```python
from build123d import *

# Parameters (mm, degrees)
F1_DEPTH = 200
F2_R     = 2
F4_DEPTH = 2
F6_D     = 5
F6_DEPTH = 2


with BuildPart() as f1:
    # F0 (on Front) → F1 (new body)
    with BuildSketch(Plane.XZ):
        Polygon((35, 0), (0, 0), (0, -345), (28, -345), (28, -295), (8, -271.164928), (8, -191.164928), (30, -130.720425), (30, -80.720425), (28, -80.720425), (28, -130.367771), (6, -190.812274), (6, -271.892869), (26, -295.72794), (26, -343), (2, -343), (2, -2), (33, -2), (33, -23), (35, -23), align=None)
    extrude(amount=F1_DEPTH)

    # F2
    f2_edges = [f1.edges().sort_by_distance(p)[0] for p in [
        (0, -100, 0),
        (35, -100, 0),
        (33, -100, -2),
        (2, -100, -2),
        (0, -100, -345),
        (2, -100, -343),
        (28, -100, -345),
        (26, -100, -343),
        (26, -100, -295.72794),
        (28, -100, -295),
        (8, -100, -271.164928),
        (6, -100, -271.892869),
        (6, -100, -190.812274),
        (8, -100, -191.164928),
        (30, -100, -130.720425),
        (28, -100, -130.367771),
    ]]
    fillet(f2_edges, radius=F2_R)

    # F3 (on face) → F4 (cut)
    with BuildSketch(Plane(origin=(0, 0, 0), x_dir=(0, -1, 0), z_dir=(-1, 0, 0))):
        with BuildLine():
            Line((70, -50), (30, -50))
            ThreePointArc((30, -50), (26.464466, -51.464466), (25, -55))
            Line((25, -55), (25, -290))
            ThreePointArc((25, -290), (26.464466, -293.535534), (30, -295))
            Line((30, -295), (70, -295))
            ThreePointArc((70, -295), (73.535534, -293.535534), (75, -290))
            Line((75, -290), (75, -55))
            ThreePointArc((75, -55), (73.535534, -51.464466), (70, -50))
        make_face()
        with BuildLine():
            ThreePointArc((175, -55), (173.535534, -51.464466), (170, -50))
            Line((170, -50), (130, -50))
            ThreePointArc((130, -50), (126.464466, -51.464466), (125, -55))
            Line((125, -55), (125, -290))
            ThreePointArc((125, -290), (126.464466, -293.535534), (130, -295))
            Line((130, -295), (170, -295))
            ThreePointArc((170, -295), (173.535534, -293.535534), (175, -290))
            Line((175, -290), (175, -55))
        make_face()
    extrude(amount=-F4_DEPTH, mode=Mode.SUBTRACT)

    # F6
    with Locations(Plane(origin=(28, 0, 0), x_dir=(0, -1, 0), z_dir=(-1, 0, 0))):
        with Locations((50, -105.367771), (150, -105.367771)):
            Hole(F6_D / 2, depth=F6_DEPTH)


solid = f1.part
```
For this review, take the finished solid that the model builds, in its own axes (mm). A direction names the side the tool comes from. Coordinates: 2 decimals unless noted, no trailing zeros. Write each loop counter-clockwise with the first axis right and the second up, starting at its lowest first coordinate (ties: lowest second). Pieces come first, ordered by that corner, then holes. Notation, with made-up numbers: (-5.75, 3.25) -> (34.25, 3.25) arc R27 ccw to (34.25, 31.25) -> close; hole circle Ø1 at (18.25, 65.25). An arc over 180 degrees is marked (long way). Put each result on its own line as item: value.
Q1. Wall thickness on L1, parallel to X at y = -106, z = -209; L2, parallel to X at y = -91, z = -115.5; L3, parallel to Z at x = 31, y = -85.5: over which ranges is each line inside the solid? List them lowest first.
From the geometry:
L1: x = 0 to 2, 6 to 8
L2: x = 0 to 2, 28 to 30
L3: z = -2 to 0
Q2. Take a section at B-B, the plane x = 17. State the section outline as (y, z) points.
From the geometry:
outline: (-200, -345) -> (0, -345) -> (0, -343) -> (-200, -343) -> close; (-200, -285) -> (0, -285) -> (0, -281.89) -> (-200, -281.89) -> close; (-200, -166.44) -> (0, -166.44) -> (0, -160.59) -> (-200, -160.59) -> close; (-200, -2) -> (0, -2) -> (0, 0) -> (-200, 0) -> close
Q3. The part is to be moulded in two halves that separate along Z. For faces 1 (the flat face through (14, -99, -345)), 2 (the flat face through (17.152, -98.6, -160.172)), 3 (the flat face through (0, -99, -170)), say which applies: +Z half, -Z half, draft (parallel to the pull), parting line (faces both ways), or undercut.
From the geometry:
face 1: -Z half
face 2: undercut
face 3: draft
Q4. Take a section at A-A, the plane z = -307.5. State the section outline as (x, y) points, then the cut area to 3 significant figures.
From the geometry:
outline: (0, -200) -> (2, -200) -> (2, 0) -> (0, 0) -> close; (26, -200) -> (28, -200) -> (28, 0) -> (26, 0) -> close
area: 800 mm2
Q5. Clearance check with flat-ended pins moving along their axes: pin 1 Ø10 at (y, z) = (-102, -248.5) entering from +X; pin 2 Ø10 at (y, z) = (-111, -294.5) entering from -X; pin 3 Ø3 at (y, z) = (-150, -105.37) entering from -X; pin 4 Ø5 at (y, z) = (-61, -129.5) entering from -X. State where each tip first meets the part, or that it passes through.
From the geometry:
pin 1: stops at x = 8
pin 2: stops at x = 0
pin 3: passes through
pin 4: stops at x = 27.41
Q6. Tool access review of faces 4 (the flat face through (26, -99, -318)), 5 (the flat face through (30, -99, -106)), 6 (the flat face through (8, -99, -232)), 7 (the flat face through (33, -99, -13)): name each direction out of +Z, -Z, +X, -X, +Y, -Y from which nothing blocks a thin tool from reaching the whole face with its end or side.
From the geometry:
face 4: +Y, -Y
face 5: -Z, +X, +Y, -Y
face 6: +X, +Y, -Y
face 7: -Z, +Y, -Y
